Verification items for the finished model (mm, model axes). Coordinates: 2 decimals unless noted, no trailing zeros. Order: outer loops, then holes, each group sorted by start corner. A loop starts at its lowest first (then second) coordinate and runs counter-clockwise, first axis right, second up. Notation, with made-up numbers: M 79,42.5 L 103,42.5 A30 cw 103,80.5 Z; hole C -37.75,-33 d6. An arc over 180 degrees is marked long. Return JSON: item names as keys, results as strings. Group by question number.
Q1. Go/stop test with a flat-tipped pin: pin 1 Ø1 at (x, y) = (-318.5, -3.5) entering from +Z. Record where the tip stops, or that it passes through.
Q2. Section check A-A, the plane x = 189.5. Enter the section's corners in (y, z).
Q3. Thickness scan on probe 1 along Y at (x, z) = (-215.9, 2.25); probe 2 along X at (y, z) = (-68.5, -2); probe 3 along Z at (x, y) = (-284, -4). Record the ranges inside material, lowest first.
from build123d import *

# Parameters (mm, degrees)
F0_W     = 901.7
F0_H     = 174.625
F1_DEPTH = 4.7625
F3_D     = 7.9375
F4_W     = 101.6
F4_H     = 101.6
F4_W_2   = 50.8
F4_H_2   = 50.8
F5_DEPTH = 0.254


with BuildPart() as f1:
    # F0 (on Top) → F1 (new body, symmetric)
    with BuildSketch(Plane.XY):
        Rectangle(F0_W, F0_H)
    extrude(amount=F1_DEPTH, both=True)

    # F3 (through all)
    with Locations(Plane.XY.offset(4.7625)):
        with Locations((-215.9, 66.675), (-215.9, 0), (-215.9, -66.675), (-431.8, 66.675), (-431.8, 0), (-431.8, -66.675), (0, 66.675), (0, 0), (0, -66.675), (215.9, 66.675), (215.9, 0), (215.9, -66.675), (431.8, -66.675), (431.8, 0), (431.8, 66.675)):
            Hole(F3_D / 2)

    # F4 (on face) → F5 (join)
    with BuildSketch(Plane.XY.offset(4.7625)):
        Rectangle(F4_W, F4_H)
        with Locations((-346.075, 0)):
            Rectangle(F4_W_2, F4_H_2)
        with Locations((346.075, 0)):
            Rectangle(F4_W_2, F4_H_2)
    extrude(amount=F5_DEPTH)


solid = f1.part
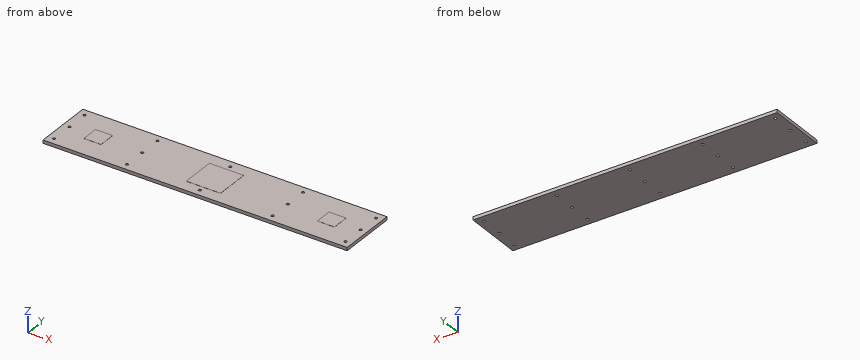
Numbers:
{
 "1": {"pin 1": "stops at z = 4.76"},
 "2": {"outline": "M -87.31,-4.76 L 87.31,-4.76 L 87.31,4.76 L -87.31,4.76 Z"},
 "3": {"probe 1": "y = -87.31 to -70.64, -62.71 to -3.97, 3.97 to 62.71, 70.64 to 87.31", "probe 2": "x = -450.85 to -435.32, -428.28 to -219.42, -212.38 to -3.52, 3.52 to 212.38, 219.42 to 428.28, 435.32 to 450.85", "probe 3": "z = -4.76 to 4.76"}
}
